The drawing under review shows one solid part. Ordinate dimensions are in mm from its lowest x, y, z. A direction names the side the tool comes from. Round coordinates to 2 decimals unless told otherwise and drop trailing zeros. Write each loop counter-clockwise with the first axis right and the second up, starting at its lowest first coordinate (ties: lowest second). Pieces come first, ordered by that corner, then holes. Notation, with made-up numbers: (-4, -15) -> (31, -15) arc R27 ccw to (31, 6) -> close; hole circle Ø11 at (-12.5, 13). An arc over 180 degrees is marked (long way). Write item = value, one per line. Start each with the question number.
Item 1: Machinability: for the marked faces 1, 2 and 3, which of the approach directions +Z, -Z, +X, -X, +Y, -Y give a long, thin tool a straight path to every point of the face, cutting with its end or side? Answer none if there is none.
Item 2: Add section C-C, the plane x = 1.2. State the section outline as (y, z) points.
Item 3: Mouldability with a two-part tool opening along X and no side actions: class the marked faces 4, 5, 6 and 7 as released by +X, released by -X, zero draft, split by the parting line, or undercut.
Item 4: To check wall thickness, follow L1, parallel to Z at x = 3.85, y = 0.25; L2, parallel to X at y = 1.7, z = 1; L3, parallel to X at y = 1.1, z = 1.5. State the ranges of each line that lie inside material, in increasing order.
Item 5: Add section D-D, the plane x = 3.95. State the section outline as (y, z) points.
Item 6: Add section A-A, the plane y = 1.25. State the section outline as (x, z) points, then the cut area to 3 significant figures.
Item 7: Add section B-B, the plane z = 3.75. State the section outline as (x, y) points (3 decimals), then the cut area to 3 significant figures.
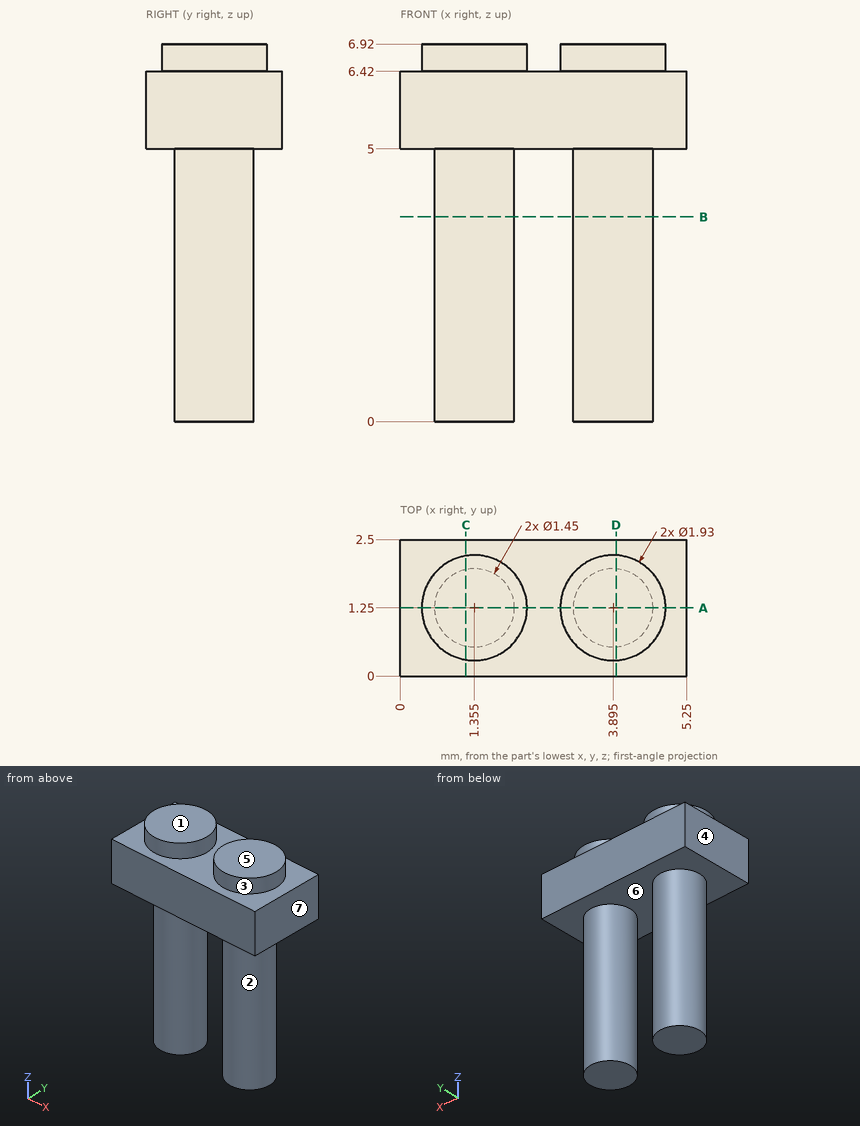
Result set:
q1.face_1 = +Z, +X, -X, +Y, -Y
q1.face_2 = -Z
q1.face_3 = +Z
q2.outline = (0, 5) -> (0.54, 5) -> (0.54, 0) -> (1.96, 0) -> (1.96, 5) -> (2.5, 5) -> (2.5, 6.42) -> (2.2, 6.42) -> (2.2, 6.92) -> (0.3, 6.92) -> (0.3, 6.42) -> (0, 6.42) -> close
q3.face_4 = released by -X
q3.face_5 = zero draft
q3.face_6 = undercut
q3.face_7 = released by +X
q4.L1 = 5 to 6.42
q4.L2 = 0.79 to 1.92, 3.33 to 4.46
q4.L3 = 0.65 to 2.06, 3.19 to 4.6
q5.outline = (0, 5) -> (0.53, 5) -> (0.53, 0) -> (1.97, 0) -> (1.97, 5) -> (2.5, 5) -> (2.5, 6.42) -> (2.21, 6.42) -> (2.21, 6.92) -> (0.29, 6.92) -> (0.29, 6.42) -> (0, 6.42) -> close
q6.outline = (0, 5) -> (0.63, 5) -> (0.63, 0) -> (2.08, 0) -> (2.08, 5) -> (3.17, 5) -> (3.17, 0) -> (4.62, 0) -> (4.62, 5) -> (5.25, 5) -> (5.25, 6.42) -> (4.86, 6.42) -> (4.86, 6.92) -> (2.93, 6.92) -> (2.93, 6.42) -> (2.32, 6.42) -> (2.32, 6.92) -> (0.39, 6.92) -> (0.39, 6.42) -> (0, 6.42) -> close
q6.area = 23.9 mm²
q7.outline = circle Ø1.45 at (1.355, 1.25); circle Ø1.45 at (3.895, 1.25)
q7.area = 3.30 mm²
